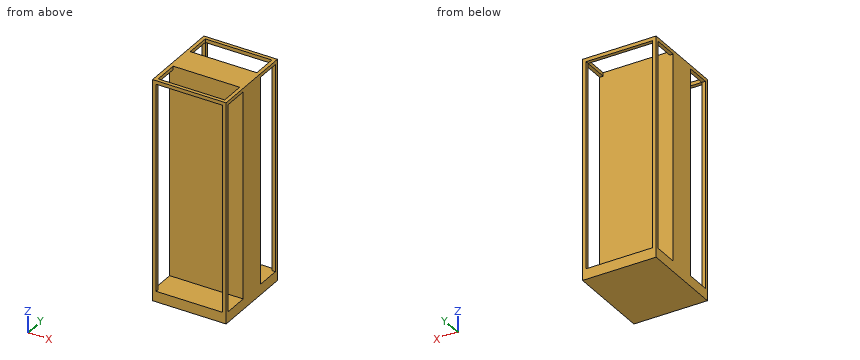
from build123d import *

# Parameters (mm, degrees)
F0_W     = 533.4
F0_H     = 203.2
F1_DEPTH = 1600.2
F2_W     = 177.8
F2_H     = 1498.6
F3_DEPTH = 533.401
F4_W     = 482.6
F4_H     = 177.8
F5_DEPTH = 76.2
F6_W     = 482.6
F6_H     = 1498.6
F7_DEPTH = 50.8


# Not quite as in the source:
# - a pattern or mirror of a feature is missing from the dataset's text; its kind, count and spacing are read off the source's solid


with BuildPart() as f1:
    # F0 (on Top) → F1 (new body)
    with BuildSketch(Plane.XY):
        with Locations((266.7, 508)):
            Rectangle(F0_W, F0_H)
        with Locations((266.7, 101.6)):
            Rectangle(F0_W, F0_H)
        with Locations((266.7, 304.8)):
            Rectangle(F0_W, F0_H)
    extrude(amount=F1_DEPTH)

    # F2 (on face) → F3 (cut, through all)
    with BuildSketch(Plane(origin=(0, 0, 0), x_dir=(0, -1, 0), z_dir=(-1, 0, 0))):
        with Locations((-495.3, 825.5)):
            Rectangle(F2_W, F2_H)
        with Locations((-114.3, 825.5)):
            Rectangle(F2_W, F2_H)
    extrude(amount=-F3_DEPTH, mode=Mode.SUBTRACT)

    # F4 (on face) → F5 (cut)
    with BuildSketch(Plane.XY.offset(1600.2)):
        with Locations((266.7, 495.3)):
            Rectangle(F4_W, F4_H)
        with Locations((266.7, 114.3)):
            Rectangle(F4_W, F4_H)
    extrude(amount=-F5_DEPTH, mode=Mode.SUBTRACT)

    # F6 (on face) → F7 (cut)
    with BuildSketch(Plane.XZ):
        with Locations((266.7, 825.5)):
            Rectangle(F6_W, F6_H)
    f7 = extrude(amount=-F7_DEPTH, mode=Mode.SUBTRACT)

    # F7_copies: F7 across plane
    add(f7.mirror(Plane.ZX.offset(304.8)), mode=Mode.SUBTRACT)


solid = f1.part
The listing builds one solid part. Answer for the finished solid, in the listing's coordinates (mm). Round coordinates to 2 decimals unless told otherwise and drop trailing zeros. Write each loop counter-clockwise with the first axis right and the second up, starting at its lowest first coordinate (ties: lowest second). Pieces come first, ordered by that corner, then holes. Notation, with made-up numbers: (26.5, 16) - (69.5, 16) arc R18 cw to (69.5, 27) - close; hole circle Ø11 at (-37, -0.5). An arc over 180 degrees is marked (long way). Use a Markdown table: item, result. Add a question column.
1. The part is cut by section A-A (z = 332). Write down the section's boundary in (x, y).
2. Consider line 1 (Y direction, x = 441.5, z = 1037.5); line 2 (Z direction, x = 456.5, y = 117). Determine where each line is inside the solid, lowest interval first.
3. The part is cut by section C-C (y = 494). Write down the section's boundary in (x, z), and give its area (3 significant figures).
4. Flat-ended cylindrical pins translate along their axes: P1, Ø1, axis at x = 232.5, z = 599.5, coming from the +Y side; P2, Ø5, axis at x = 294, z = 943, coming from the -Y side. Find the tip coordinate at first contact, or state that the pin passes through.
5. The part is cut by section B-B (x = 420.5). Write down the section's boundary in (y, z), and give its area (3 significant figures).
Reported:
| question | item | result |
|---|---|---|
| 1 | outline | (0, 0) - (25.4, 0) - (25.4, 25.4) - (0, 25.4) - close; (0, 203.2) - (533.4, 203.2) - (533.4, 406.4) - (0, 406.4) - close; (0, 584.2) - (25.4, 584.2) - (25.4, 609.6) - (0, 609.6) - close; (508, 0) - (533.4, 0) - (533.4, 25.4) - (508, 25.4) - close; (508, 584.2) - (533.4, 584.2) - (533.4, 609.6) - (508, 609.6) - close |
| 2 | line 1 | 203.2 to 406.4 |
| 2 | line 2 | 0 to 76.2 |
| 3 | outline | (0, 0) - (533.4, 0) - (533.4, 76.2) - (0, 76.2) - close; (0, 1574.8) - (25.4, 1574.8) - (25.4, 1600.2) - (0, 1600.2) - close; (508, 1574.8) - (533.4, 1574.8) - (533.4, 1600.2) - (508, 1600.2) - close |
| 3 | area | 41,900 mm^2 |
| 4 | P1 | y = 406.4 |
| 4 | P2 | y = 203.2 |
| 5 | outline | (0, 0) - (609.6, 0) - (609.6, 76.2) - (406.4, 76.2) - (406.4, 1600.2) - (203.2, 1600.2) - (203.2, 76.2) - (0, 76.2) - close; (0, 1574.8) - (25.4, 1574.8) - (25.4, 1600.2) - (0, 1600.2) - close; (584.2, 1574.8) - (609.6, 1574.8) - (609.6, 1600.2) - (584.2, 1600.2) - close |
| 5 | area | 357,000 mm^2 |
